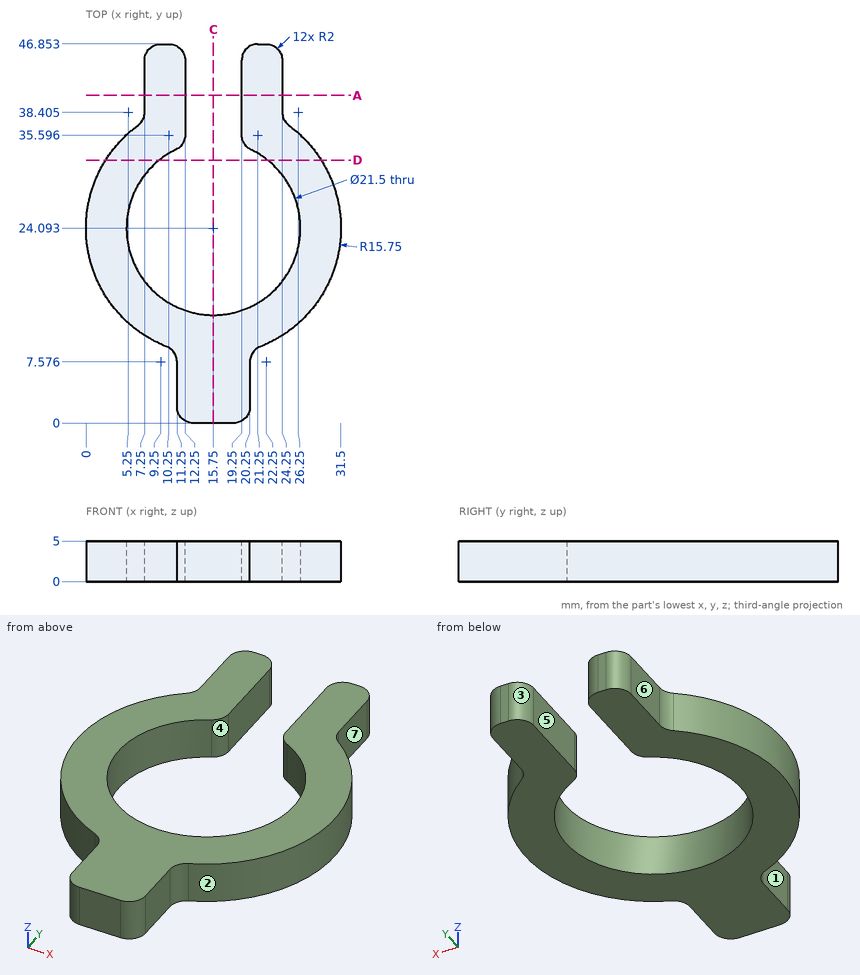
Check sheet for the drawn part. Datum: minimum x, y, z corner. Units: mm. A direction names the side the tool comes from. Round coordinates to 2 decimals unless told otherwise and drop trailing zeros. Write each loop counter-clockwise with the first axis right and the second up, starting at its lowest first coordinate (ties: lowest second). Pieces come first, ordered by that corner, then holes. Notation, with made-up numbers: (4, 3.25) -> (25, 3.25) arc R12 ccw to (25, 9.25) -> close; hole circle Ø5 at (83.25, 30). An arc over 180 degrees is marked (long way). Write each question's results on one line, items separated by ' | '.
Q1. Thickness scan on probe 1 along X at (y, z) = (41, 4.1); probe 2 along X at (y, z) = (45, 2.55) (1 decimal); probe 3 along Y at (x, z) = (19.5, 4.25) (1 decimal). Record the ranges inside material, lowest first.
Derived:
probe 1: x = 7.25 to 12.25, 19.25 to 24.25 | probe 2: x = 7.3 to 12.2, 19.3 to 24.2 | probe 3: y = 0.4 to 14, 34.6 to 45.8
Q2. Sectioned sample at C-C, the plane x = 15.75. Record the boundary of the cut face in (y, z).
Derived:
outline: (0, 0) -> (13.34, 0) -> (13.34, 5) -> (0, 5) -> close
Q3. Sectioned sample at D-D, the plane y = 32.5. Record the boundary of the cut face in (x, z).
Derived:
outline: (2.43, 0) -> (9.05, 0) -> (9.05, 5) -> (2.43, 5) -> close; (22.45, 0) -> (29.07, 0) -> (29.07, 5) -> (22.45, 5) -> close
Q4. Access from +Z, -Z, +X, -X, +Y, -Y to the whole of each face (thin tool, end or side, straight path). Record for the marked faces 4, 5, 6 and 7.
Derived:
face 4: +Z, -Z | face 5: +Z, -Z, +Y | face 6: +Z, -Z, -X, +Y | face 7: +Z, -Z, +X, +Y
Q5. Go/stop test with flat-tipped pins: pin 1 Ø17 at (x, y) = (15.75, 24.09) entering from -Z; pin 2 Ø3 at (x, z) = (27.5, 4) entering from -Y (1 decimal); pin 3 Ø2.5 at (y, z) = (39.5, 1.5) entering from -X; pin 4 Ø1 at (x, z) = (25, 2.5) entering from +Y (1 decimal). Record where each tip stops, or that it passes through.
Derived:
pin 1: passes through | pin 2: stops at y = 12.1 | pin 3: stops at x = 7.24 | pin 4: stops at y = 37.4
Q6. Draft check along X on the marked faces 1, 2 and 3. Enter one of: released by +X, released by -X, zero draft, split by the parting line, or undercut.
Derived:
face 1: released by -X | face 2: released by +X | face 3: undercut
Q7. Sectioned sample at A-A, the plane y = 40.5. Record the boundary of the cut face in (x, z).
Derived:
outline: (7.25, 0) -> (12.25, 0) -> (12.25, 5) -> (7.25, 5) -> close; (19.25, 0) -> (24.25, 0) -> (24.25, 5) -> (19.25, 5) -> close
